Source: CAD feature listing. Evaluate the final solid. Frame: model axes, mm. A direction names the side the tool comes from. Round coordinates to 2 decimals unless told otherwise and drop trailing zeros. Loops run counter-clockwise (first coordinate to the right, second up) from the corner with the lowest first, then second, coordinate; pieces in that order, holes last. Notation, with made-up numbers: (68.5, 21.25) -> (126.5, 21.25) arc R28 ccw to (126.5, 54.25) -> close; hole circle Ø5 at (-15, -28.5). An arc over 180 degrees is marked (long way). Put each result on its own line as item: value. Start each with the question number.
1. Draft query along Z for faces 3 (the flat face through (46.625, 1, 1)), 4 (the cylindrical face through (13.77, 3.99, -22.14)), 5 (the flat face through (1, 1, -62.25)). Return one class per face: pulls with the +Z half, pulls with the -Z half, needs draft (parallel to the pull), parting line crosses it, or undercut.
2. Contact query for flat-ended pins moving along their axis: pin 1 (2.5 mm diameter, centred on x = 2.88, z = -44.83, fed in from +Y); pin 2 (8 mm diameter, centred on x = -36.5, z = -44.5, fed in from +Y); pin 3 (1.6 mm diameter, centred on x = -45.5, y = 1, fed in from +Z); pin 4 (0.8 mm diameter, centred on x = -46, y = 1, fed in from -Z). Output: stop coordinate, or through.
3. Cut plane B-B (x = 19.5). Return the cut outline in (y, z), then the cut area to 4 significant figures.
4. Set-up query: faces 1 (the flat face through (-1, 0, -1)), 2 (the flat face through (13, 5, 19)). Return all of +Z, -Z, +X, -X, +Y, -Y with unobstructed straight access to the full face (end or side cutting, diameter ignored); none if empty.
5. Cut plane A-A (z = 54.5). Return the cut outline in (x, y) (3 decimals).
6. Material intervals for L1, parallel to Y at x = -39, z = -10; L2, parallel to Z at x = -23.5, y = 5.75, sorted ascending.
```python
from build123d import *

# Parameters (mm, degrees)
SKETCH1_W           = 93.25
SKETCH1_H           = 124.5
BOSS_EXTRUDE1_DEPTH = 3
SKETCH2_R           = 1.45
CUT_EXTRUDE1_DEPTH  = 78.832853764
SKETCH6_R           = 2
SKETCH6_R_2         = 1
BOSS_EXTRUDE4_DEPTH = 2
SKETCH7_R           = 1
BOSS_EXTRUDE5_DEPTH = 4
SKETCH8_R           = 1.5
CUT_EXTRUDE2_DEPTH  = 3
CUT_EXTRUDE3_DEPTH  = 3
CUT_EXTRUDE4_DEPTH  = 3


with BuildPart() as part:
    # Sketch1 → Boss-Extrude1 (new body)
    with BuildSketch(Plane(origin=(0, 0, 0), x_dir=(1, 0, 0), z_dir=(0, 1, 0))):
        Rectangle(SKETCH1_W, SKETCH1_H)
    extrude(amount=BOSS_EXTRUDE1_DEPTH)

    # Sketch2 → Cut-Extrude1 (cut, through all)
    with BuildSketch(Plane(origin=(0, 3, 0), x_dir=(1, 0, 0), z_dir=(0, 1, 0))):
        with Locations(Location((-45.125, 60.75, 0), (0, 0, 270))):
            Circle(SKETCH2_R)
        with Locations(Location((-45.125, -60.75, 0), (0, 0, 270))):
            Circle(SKETCH2_R)
    extrude(amount=-CUT_EXTRUDE1_DEPTH, mode=Mode.SUBTRACT)

    # Sketch6 → Boss-Extrude4 (add)
    # profile 1 of 3: a face of its own
    with BuildSketch(Plane(origin=(0, 3, 0), x_dir=(1, 0, 0), z_dir=(0, 1, 0))):
        with Locations(Location((-24.225, -7.367286263, 0), (0, 0, 90))):
            Circle(SKETCH6_R)
        with Locations(Location((-24.225, -7.367286263, 0), (0, 0, 270))):
            Circle(SKETCH6_R_2, mode=Mode.SUBTRACT)
    # profile 2 of 3: a face of its own
    with BuildSketch(Plane(origin=(0, 3, 0), x_dir=(1, 0, 0), z_dir=(0, 1, 0))):
        with Locations(Location((14.375, 20.232713737, 0), (0, 0, 90))):
            Circle(SKETCH6_R)
        with Locations(Location((14.375, 20.232713737, 0), (0, 0, 270))):
            Circle(SKETCH6_R_2, mode=Mode.SUBTRACT)
    # profile 3 of 3: a face of its own
    with BuildSketch(Plane(origin=(0, 3, 0), x_dir=(1, 0, 0), z_dir=(0, 1, 0))):
        with Locations(Location((14.375, -19.567286263, 0), (0, 0, 90))):
            Circle(SKETCH6_R)
        with Locations(Location((14.375, -19.567286263, 0), (0, 0, 270))):
            Circle(SKETCH6_R_2, mode=Mode.SUBTRACT)
    extrude(amount=BOSS_EXTRUDE4_DEPTH)

    # Sketch7 → Boss-Extrude5 (add)
    with BuildSketch(Plane(origin=(0, 3, 0), x_dir=(1, 0, 0), z_dir=(0, 1, 0))):
        with Locations(Location((-24.225, -7.367286263, 0), (0, 0, 270))):
            Circle(SKETCH7_R)
        with Locations(Location((14.375, 20.232713737, 0), (0, 0, 270))):
            Circle(SKETCH7_R)
        with Locations(Location((14.375, -19.567286263, 0), (0, 0, 270))):
            Circle(SKETCH7_R)
    extrude(amount=BOSS_EXTRUDE5_DEPTH)

    # Sketch8 → Cut-Extrude2 (cut)
    with BuildSketch(Plane(origin=(0, 3, 0), x_dir=(1, 0, 0), z_dir=(0, 1, 0))):
        with Locations(Location((2.875, 44.832713737, 0), (0, 0, 270))):
            Circle(SKETCH8_R)
        with Locations(Location((-41.625, 0.332713737, 0), (0, 0, 270))):
            Circle(SKETCH8_R)
        with Locations(Location((2.875, -44.167286263, 0), (0, 0, 270))):
            Circle(SKETCH8_R)
    extrude(amount=-CUT_EXTRUDE2_DEPTH, mode=Mode.SUBTRACT)

    # Sketch9 → Cut-Extrude3 (cut)
    with BuildSketch(Plane(origin=(0, 3, 0), x_dir=(1, 0, 0), z_dir=(0, 1, 0))):
        with BuildLine():
            Line((-45.125, 59.3), (-46.625, 59.3))
            Line((-46.625, 59.3), (-46.625, 62.25))
            Line((-46.625, 62.25), (-43.675, 62.25))
            Line((-43.675, 62.25), (-43.675, 60.75))
            ThreePointArc((-43.675, 60.75), (-44.099695167, 59.724695167), (-45.125, 59.3))
        make_face()
    extrude(amount=-CUT_EXTRUDE3_DEPTH, mode=Mode.SUBTRACT)

    # Sketch10 → Cut-Extrude4 (cut)
    with BuildSketch(Plane(origin=(0, 3, 0), x_dir=(1, 0, 0), z_dir=(0, 1, 0))):
        with BuildLine():
            Line((-45.125, -59.3), (-46.625, -59.3))
            Line((-46.625, -59.3), (-46.625, -62.25))
            Line((-46.625, -62.25), (-43.675, -62.25))
            Line((-43.675, -62.25), (-43.675, -60.75))
            ThreePointArc((-43.675, -60.75), (-44.099695167, -59.724695167), (-45.125, -59.3))
        make_face()
    extrude(amount=-CUT_EXTRUDE4_DEPTH, mode=Mode.SUBTRACT)


solid = part.part
```
Solution:
1. face 3: needs draft
1. face 4: undercut
1. face 5: pulls with the -Z half
2. pin 1: passes through
2. pin 2: stops at y = 3
2. pin 3: stops at z = 59.36
2. pin 4: stops at z = -59.3
3. outline: (0, -62.25) -> (3, -62.25) -> (3, 62.25) -> (0, 62.25) -> close
3. area: 373.5 mm^2
4. face 1: +Z, -Z, +X, -X, -Y
4. face 2: +Y
5. outline: (-46.625, 0) -> (46.625, 0) -> (46.625, 3) -> (-46.625, 3) -> close
6. L1: y = 0 to 3
6. L2: z = 6.68 to 8.06
